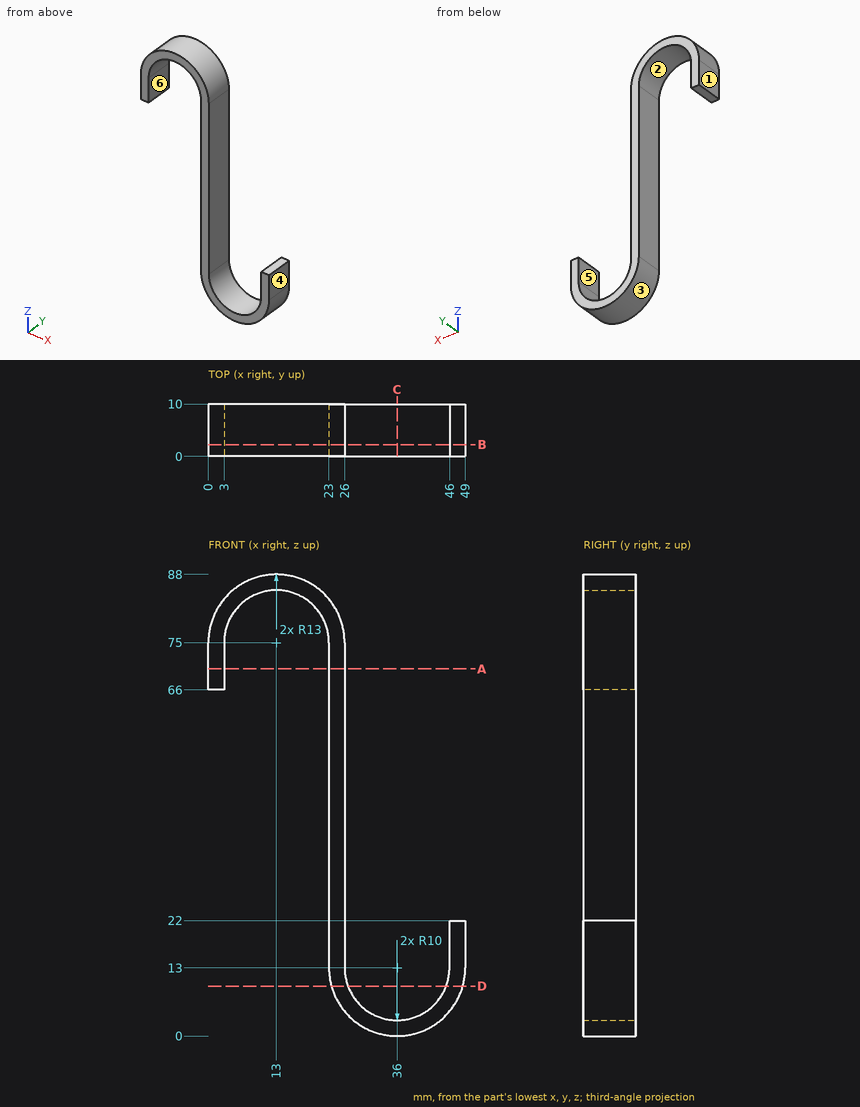
Could you check a few things on this drawing? It's one solid part, dimensions in mm from its lowest x, y, z. A direction names the side the tool comes from. Coordinates: 2 decimals unless noted, no trailing zeros. Write each loop counter-clockwise with the first axis right and the second up, starting at its lowest first coordinate (ties: lowest second). Pieces come first, ordered by that corner, then holes.
Q1. Imagine slicing it at D-D, the plane z = 9.5. List the corners of the cut face in (x, y) for me.
Results found:
outline: (23.48, 0) - (26.63, 0) - (26.63, 10) - (23.48, 10) - close; (45.37, 0) - (48.52, 0) - (48.52, 10) - (45.37, 10) - close
Q2. Imagine slicing it at B-B, the plane y = 2.25. List the corners of the cut face in (x, z) for me, plus the area to 3 significant figures.
Results found:
outline: (0, 66) - (3, 66) - (3, 75) arc R10 cw to (23, 75) - (23, 13) arc R13 ccw to (49, 13) - (49, 22) - (46, 22) - (46, 13) arc R10 cw to (26, 13) - (26, 75) arc R13 ccw to (0, 75) - close
area: 457 mm2
Q3. If we mould it in two halves opening along X, with no side actions, what happens to the marked faces 1, 2 and 3? For each: +X half, -X half, draft (parallel to the pull), parting line (faces both ways), or undercut.
Results found:
face 1: -X half
face 2: undercut
face 3: parting line
Q4. For P1, Ø5, axis at x = 14, y = 5, coming from the -Z side; P2, Ø2.5, axis at y = 4, z = 69.5, coming from the +X side; P3, Ø2.5, axis at x = 1.5, y = 4, coming from the -Z side, each with a flat end and sliding along its axis, tell me the tip position at first contact or that it passes through.
Results found:
P1: stops at z = 84.37
P2: stops at x = 26
P3: stops at z = 66
Q5. Imagine slicing it at C-C, the plane x = 36. List the corners of the cut face in (y, z) for me, plus the area to 3 significant figures.
Results found:
outline: (0, 0) - (10, 0) - (10, 3) - (0, 3) - close
area: 30.0 mm2
Q6. Which directions (+Z, -Z, +X, -X, +Y, -Y) give clear straight access to the entire face, cutting with the end or side of a thin tool? Please do the marked faces 4, 5 and 6.
Results found:
face 4: +Z, -Z, +X, +Y, -Y
face 5: +Z, +Y, -Y
face 6: -Z, +Y, -Y
Q7. Imagine slicing it at A-A, the plane z = 70. List the corners of the cut face in (x, y) for me.
Results found:
outline: (0, 0) - (3, 0) - (3, 10) - (0, 10) - close; (23, 0) - (26, 0) - (26, 10) - (23, 10) - close
Q8. Please list where these lines run through material, in increasing order: L1, parallel to X at y = 2.25, z = 73; L2, parallel to X at y = 8.5, z = 18.5; L3, parallel to X at y = 5.75, z = 54.5.
Results found:
L1: x = 0 to 3, 23 to 26
L2: x = 23 to 26, 46 to 49
L3: x = 23 to 26
